For this review, take the finished solid that the model builds, in its own axes (mm). Face numbers are marked on the shaded views. A direction names the side the tool comes from. Round coordinates to 2 decimals unless told otherwise and drop trailing zeros. Order: outer loops, then holes, each group sorted by start corner. A loop starts at its lowest first (then second) coordinate and runs counter-clockwise, first axis right, second up. Notation, with made-up numbers: (79.5, -15) - (111.5, -15) arc R18 cw to (111.5, 3) - close; hole circle Ø4 at (66.25, 29). An arc over 180 degrees is marked (long way). One line per item, written item: value.
```python
from build123d import *

# Parameters (mm, degrees)
F0_R     = 41.79738
F1_DEPTH = 12.7
F2_R     = 12.959367
F3_DEPTH = 50.8
F4_R     = 6.983691
F5_DEPTH = 12.7
F8_D     = 7.62
F10_D    = 12.7


with BuildPart() as f1:
    # F0 (on Top) → F1 (new body)
    with BuildSketch(Plane.XY):
        Circle(F0_R)
    extrude(amount=F1_DEPTH)

    # F2 (on face) → F3 (join)
    with BuildSketch(Plane.XY.offset(12.7)):
        Circle(F2_R)
    extrude(amount=F3_DEPTH)

    # F4 (on face) → F5 (join)
    with BuildSketch(Plane.XY.offset(63.5)):
        Circle(F4_R)
    extrude(amount=F5_DEPTH)

    # F8 (through all)
    with Locations(Plane.XY.offset(76.2)):
        with Locations((0, 0)):
            Hole(F8_D / 2)

    # F10 (through all)
    with Locations(Plane.XY.offset(12.7)):
        with Locations((0, -26.591428), (-24.934307, 0), (24.870217, 0), (0, 24.461392)):
            Hole(F10_D / 2)


solid = f1.part
```
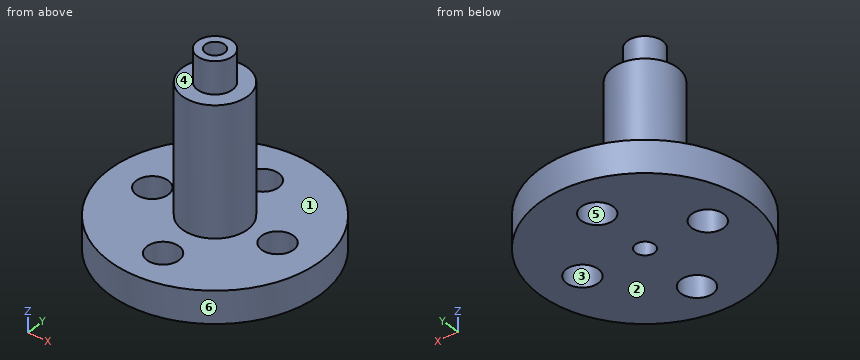
Item 1: Take a section at C-C (z = 15). Write out the cut boundary in (x, y).
Returned:
outline: circle Ø25.92 at (0, 0); hole circle Ø7.62 at (0, 0)
Item 2: Take a section at A-A (x = 0). Write out the cut boundary in (y, z), plus the area to 3 significant figures.
Returned:
outline: (-41.8, 0) - (-32.94, 0) - (-32.94, 12.7) - (-41.8, 12.7) - close; (-20.24, 0) - (-3.81, 0) - (-3.81, 76.2) - (-6.98, 76.2) - (-6.98, 63.5) - (-12.96, 63.5) - (-12.96, 12.7) - (-20.24, 12.7) - close; (3.81, 0) - (18.11, 0) - (18.11, 12.7) - (12.96, 12.7) - (12.96, 63.5) - (6.98, 63.5) - (6.98, 76.2) - (3.81, 76.2) - close; (30.81, 0) - (41.8, 0) - (41.8, 12.7) - (30.81, 12.7) - close
area: 1,650 mm^2
Item 3: Take a section at D-D (x = 27.5). Write out the cut boundary in (y, z), plus the area to 3 significant figures.
Returned:
outline: (-31.48, 0) - (-5.78, 0) - (-5.78, 12.7) - (-31.48, 12.7) - close; (5.78, 0) - (31.48, 0) - (31.48, 12.7) - (5.78, 12.7) - close
area: 653 mm^2
Item 4: Wall thickness on line 1 (Y direction, x = 0, z = 3.25); line 2 (Y direction, x = 0, z = 18.5); line 3 (Z direction, x = -3.5, y = -10): over which ranges is each line inside the solid? List them lowest first.
Returned:
line 1: -41.8 to -32.94, -20.24 to -3.81, 3.81 to 18.11, 30.81 to 41.8
line 2: -12.96 to -3.81, 3.81 to 12.96
line 3: 0 to 63.5
Item 5: Take a section at B-B (y = 0). Write out the cut boundary in (x, z), plus the area to 3 significant figures.
Returned:
outline: (-41.8, 0) - (-31.28, 0) - (-31.28, 12.7) - (-41.8, 12.7) - close; (-18.58, 0) - (-3.81, 0) - (-3.81, 76.2) - (-6.98, 76.2) - (-6.98, 63.5) - (-12.96, 63.5) - (-12.96, 12.7) - (-18.58, 12.7) - close; (3.81, 0) - (18.52, 0) - (18.52, 12.7) - (12.96, 12.7) - (12.96, 63.5) - (6.98, 63.5) - (6.98, 76.2) - (3.81, 76.2) - close; (31.22, 0) - (41.8, 0) - (41.8, 12.7) - (31.22, 12.7) - close
area: 1,650 mm^2
Item 6: For P1, Ø2, axis at x = -1.5, z = 11.5, coming from the -Y side; P2, Ø10, axis at x = 0, y = -26.59, coming from the -Z side; P3, Ø3, axis at x = 5, y = 29, coming from the +Z side; P4, Ø1.5, axis at x = -12.5, z = 55, coming from the +Y side, all flat-tipped, find the tip position at first contact; note any pin that passes through.
Returned:
P1: y = -41.79
P2: through
P3: z = 12.7
P4: y = 5.47
Item 7: The part is to be moulded in two halves that separate along X. For the marked faces 3, 4, 5 and 6, say which applies: +X half, -X half, draft (parallel to the pull), parting line (faces both ways), or undercut.
Returned:
face 3: undercut
face 4: draft
face 5: undercut
face 6: parting line
Item 8: Machinability: for the marked faces 1 and 2, which of the approach directions +Z, -Z, +X, -X, +Y, -Y give a long, thin tool a straight path to every point of the face, cutting with its end or side? Answer none if there is none.
Returned:
face 1: +Z
face 2: -Z, +X, -X, +Y, -Y
